Geometry: final body of the model. Coordinates: model frame, mm. A direction names the side the tool comes from. Round coordinates to 2 decimals unless told otherwise and drop trailing zeros. Loops run counter-clockwise (first coordinate to the right, second up) from the corner with the lowest first, then second, coordinate; pieces in that order, holes last. Notation, with made-up numbers: M 73,-28.75 L 113,-28.75 A9 cw 113,-14.75 Z; hole C 29.25,2.5 d4. An arc over 180 degrees is marked long. Answer as a JSON object with one key per item and string values.
from build123d import *

# Parameters (mm, degrees)
F0_W     = 200
F0_H     = 50
F1_DEPTH = 35
F2_R     = 5
F3_T     = -2.5


with BuildPart() as f1:
    # F0 (on Top) → F1 (new body)
    with BuildSketch(Plane.XY):
        with Locations((-100, 25)):
            Rectangle(F0_W, F0_H)
    extrude(amount=F1_DEPTH)

    # F2
    f2_edges = [f1.edges().sort_by_distance(p)[0] for p in [
        (0, 0, 17.5),
        (0, 25, 35),
        (0, 50, 17.5),
        (-100, 50, 35),
        (-100, 0, 35),
        (-200, 0, 17.5),
        (-200, 25, 35),
        (-200, 50, 17.5),
    ]]
    fillet(f2_edges, radius=F2_R)

    # F3
    f3_openings = [f1.faces().sort_by_distance(p)[0] for p in [
        (-100, 25, 0),
    ]]
    offset(amount=F3_T, openings=f3_openings)


solid = f1.part
1) Section query C-C (y = 32). Return the cut outline in (x, z), and give its area (3 significant figures).
Results:
{"outline": "M -200,0 L -197.5,0 L -197.5,30 A2.5 cw -195,32.5 L -5,32.5 A2.5 cw -2.5,30 L -2.5,0 L 0,0 L 0,30 A5 ccw -5,35 L -195,35 A5 ccw -200,30 Z", "area": "654 mm2"}
2) Ray query, line 1 (X direction, y = 41, z = 3); line 2 (Y direction, x = -19, z = 19); line 3 (Z direction, x = -168, y = 42). Return the intervals inside material, ascending.
Results:
{"line 1": "-200 to -197.5, -2.5 to 0", "line 2": "0 to 2.5, 47.5 to 50", "line 3": "32.5 to 35"}
3) Reachability of faces 1 (the cylindrical face through (-199, 2, 15)), 2 (the flat face through (-101, 47.5, 15)) from +Z, -Z, +X, -X, +Y, -Y: full face, straight path, thin tool, end or side. Return the list, or none.
Results:
{"face 1": "+Z, -Z, -X, -Y", "face 2": "-Z"}
4) Pull-direction query (X, two-part tool) for faces 3 (the cylindrical face through (-199, 25, 33)), 4 (the flat face through (-101, 0, 15)), 5 (the flat face through (-197.5, 25, 15)); classes: +X half, -X half, draft (parallel to the pull), parting line (faces both ways), or undercut.
Results:
{"face 3": "-X half", "face 4": "draft", "face 5": "undercut"}
5) Section query A-A (z = 3). Return the cut outline in (x, y).
Results:
{"outline": "M -200,5 A5 ccw -195,0 L -5,0 A5 ccw 0,5 L 0,45 A5 ccw -5,50 L -195,50 A5 ccw -200,45 Z; hole M -197.5,5 A2.5 ccw -195,2.5 L -5,2.5 A2.5 ccw -2.5,5 L -2.5,45 A2.5 ccw -5,47.5 L -195,47.5 A2.5 ccw -197.5,45 Z"}
6) Section query B-B (x = -169). Return the cut outline in (y, z).
Results:
{"outline": "M 0,0 L 2.5,0 L 2.5,30 A2.5 cw 5,32.5 L 45,32.5 A2.5 cw 47.5,30 L 47.5,0 L 50,0 L 50,30 A5 ccw 45,35 L 5,35 A5 ccw 0,30 Z"}
7) Pin query (flat end, axial travel): P1, Ø6, axis at x = -112.5, y = 21, coming from the -Z side. Return the tip coordinate at first contact, or that it passes through.
Results:
{"P1": "z = 32.5"}
